```python
from build123d import *

# Parameters (mm, degrees)
SKETCH3_R          = 1.25
CUT_EXTRUDE1_DEPTH = 6


with BuildPart() as part:
    # Sketch2 → Revolve1 (revolve)
    with BuildSketch(Plane.XY, mode=Mode.PRIVATE) as revolve1_sk:
        Polygon((-12, 0), (-5, 0), (-5, 4), (-4.5, 4), (-4.5, 14), (-5, 14), (-5, 18), (-6, 18), (-6, 9), (-6.75, 9), (-6.75, 3), (-12, 3), align=None)
    revolve(revolve1_sk.sketch.rotate(Axis((0, 0, 0), (0, 1, 0)), 270), axis=Axis((0, 0, 0), (0, 1, 0)))

    # Sketch3 → Cut-Extrude1 (cut)
    with BuildSketch(Plane.XZ):
        with Locations(Location((0, 8, 0), (0, 0, 270))):
            Circle(SKETCH3_R)
        with Locations(Location((9.5, 0, 0), (0, 0, 270))):
            Circle(SKETCH3_R)
        with Locations(Location((0, -8, 0), (0, 0, 270))):
            Circle(SKETCH3_R)
        with Locations(Location((-9.5, 0, 0), (0, 0, 270))):
            Circle(SKETCH3_R)
    extrude(amount=-CUT_EXTRUDE1_DEPTH, mode=Mode.SUBTRACT)


solid = part.part
```
CAD build for the part. Positions are in the model's coordinates, mm. A direction names the side the tool comes from. Round coordinates to 2 decimals unless told otherwise and drop trailing zeros. Write each loop counter-clockwise with the first axis right and the second up, starting at its lowest first coordinate (ties: lowest second). Pieces come first, ordered by that corner, then holes. Notation, with made-up numbers: (46, 8.5) - (67, 8.5) arc R17 ccw to (67, 18.5) - close; hole circle Ø6 at (30.25, 4.25). An arc over 180 degrees is marked (long way). Write item = value, one per line. Start each with the question number.
Q1. Band-saw the part on C-C (x = 3.75). Give the cut face in (y, z), then the cut area to 3 significant figures.
Q2. Probe L1, parallel to X at y = 1.9, z = 0; L2, parallel to X at y = 7, z = 0; L3, parallel to X at y = 17.05, z = 0. List the from-to ranges inside material, lowest first. Write a range as from..to.
Q3. Drop flat-ended pins along their axis: pin 1 (7 mm diameter, centred on x = -3, z = 1, fed in from +Y); pin 2 (6 mm diameter, centred on x = 0, z = 0, fed in from +Y); pin 3 (10 mm diameter, centred on y = 12.5, z = 3, fed in from -X); pin 4 (4 mm diameter, centred on x = 9.5, z = 0, fed in from +Y). Give the stop position or say it passes through.
Q4. Mould opens along X. For faces 1 (the flat face through (-0.2, 0, -5.2)), 2 (the cylindrical face through (-3.604, 1.479, -11.446)), 3 (the cylindrical face through (-8.26, 1.48, 0.16)) say: pulls with the +X half, pulls with the -X half, needs draft (parallel to the pull), parting line crosses it, or undercut.
Q5. Band-saw the part on D-D (y = 15). Give the cut face in (x, z), then the cut area to 3 significant figures.
Q6. Band-saw the part on A-A (z = 0). Count the separate pieces of the cut face and the enclosed holes in it, then the cut area to 3 significant figures.
Q7. Band-saw the part on B-B (z = -4). Give the cut face in (x, y).
Q8. Which spindle directions (+Z, -Z, +X, -X, +Y, -Y) get a long thin tool onto all of the face, cutting with end or side? Do faces 4 (the cylindrical face through (4.88, 2.03, 1.08)), 5 (the cylindrical face through (0.05, 1.48, -6.75)), 6 (the cylindrical face through (6.59, 5.96, 1.46)). Say none if no direction does.
Answers below:
q1.outline = (0, -11.4) - (3, -11.4) - (3, -5.61) - (9, -5.61) - (9, -4.68) - (18, -4.68) - (18, -3.31) - (14, -3.31) - (14, -2.49) - (4, -2.49) - (4, -3.31) - (0, -3.31) - close; (0, 3.31) - (4, 3.31) - (4, 2.49) - (14, 2.49) - (14, 3.31) - (18, 3.31) - (18, 4.68) - (9, 4.68) - (9, 5.61) - (3, 5.61) - (3, 11.4) - (0, 11.4) - close
q1.area = 117 mm2
q2.L1 = -12..-10.75, -8.25..-5, 5..8.25, 10.75..12
q2.L2 = -6.75..-4.5, 4.5..6.75
q2.L3 = -6..-5, 5..6
q3.pin_1 = 18
q3.pin_2 = through
q3.pin_3 = -6.75
q3.pin_4 = 3
q4.face_1 = needs draft
q4.face_2 = parting line crosses it
q4.face_3 = undercut
q5.outline = circle Ø12 at (0, 0); hole circle Ø10 at (0, 0)
q5.area = 34.6 mm2
q6.separate_pieces = 4
q6.enclosed_holes = 0
q6.area = 76.0 mm2
q7.outline = (-11.31, 0) - (-3, 0) - (-3, 4) - (-2.06, 4) - (-2.06, 14) - (-3, 14) - (-3, 18) - (-4.47, 18) - (-4.47, 9) - (-5.44, 9) - (-5.44, 3) - (-11.31, 3) - close; (2.06, 4) - (3, 4) - (3, 0) - (11.31, 0) - (11.31, 3) - (5.44, 3) - (5.44, 9) - (4.47, 9) - (4.47, 18) - (3, 18) - (3, 14) - (2.06, 14) - close
q8.face_4 = -Y
q8.face_5 = +Y, -Y
q8.face_6 = +Y
